```python
from build123d import *

# Parameters (mm, degrees)
CROQUIS1_W              = 300
CROQUIS1_H              = 320
CROQUIS1_W_2            = 280
CROQUIS1_H_2            = 300
SALIENTE_EXTRUIR1_DEPTH = 50
CROQUIS2_R              = 4
CROQUIS2_R_2            = 11
CORTAR_EXTRUIR1_DEPTH   = 321
SKETCH1_R               = 1.09
CUT_EXTRUDE1_DEPTH      = 10


with BuildPart() as part:
    # Croquis1 → Saliente-Extruir1 (new body)
    with BuildSketch(Plane(origin=(0, 0, 0), x_dir=(1, 0, 0), z_dir=(0, 1, 0))):
        Rectangle(CROQUIS1_W, CROQUIS1_H)
        Rectangle(CROQUIS1_W_2, CROQUIS1_H_2, mode=Mode.SUBTRACT)
    extrude(amount=SALIENTE_EXTRUIR1_DEPTH)

    # Croquis2 → Cortar-Extruir1 (cut, through all)
    with BuildSketch(Plane.XY.offset(160)):
        with Locations((-87, 38.5)):
            Circle(CROQUIS2_R)
        with Locations((0, 35.5)):
            Circle(CROQUIS2_R_2)
        with Locations((87, 38.5)):
            Circle(CROQUIS2_R)
    extrude(amount=-CORTAR_EXTRUIR1_DEPTH, mode=Mode.SUBTRACT)

    # Sketch1 → Cut-Extrude1 (cut)
    with BuildSketch(Plane(origin=(0, 0, -160), x_dir=(-1, 0, 0), z_dir=(0, 0, -1))):
        with Locations((0, 13.579689783)):
            Circle(SKETCH1_R)
        with Locations((-21.920310217, 35.5)):
            Circle(SKETCH1_R)
        with Locations((21.920310217, 35.5)):
            Circle(SKETCH1_R)
    extrude(amount=-CUT_EXTRUDE1_DEPTH, mode=Mode.SUBTRACT)


solid = part.part
```
Could you check a few things on this model? Use its own coordinates, in mm. A direction names the side the tool comes from. Round coordinates to 2 decimals unless told otherwise and drop trailing zeros. Loops run counter-clockwise (first coordinate to the right, second up) from the corner with the lowest first, then second, coordinate; pieces in that order, holes last.
Q1. For P1, Ø1.7, axis at x = 0, y = 13.58, coming from the -Z side, with a flat end and sliding along its axis, tell me the tip position at first contact or that it passes through.
Q2. I want a section at B-B (x = -87). Write out the boundary of the cut face in (y, z), and give its area (3 significant figures).
Q3. I want a section at D-D (y = 7). Write out the boundary of the cut face in (x, z), and give its area (3 significant figures).
Q4. On a 3-axis mill with a long thin cutter (end or side, diameter ignored), from which of +Z, -Z, +X, -X, +Y, -Y can I reach the whole of each face in a straight line? I mean faces 5 (the flat face through (-2, 19, 160)), 6 (the flat face through (140, 25, 2)). Say none if no direction works.
Q5. Please list where these lines run through material, in increasing order: L1, parallel to Y at x = 0, z = -153; L2, parallel to X at y = 38.5, z = 93; L3, parallel to Z at x = 110, y = 19.
Q6. Thinking about a two-plate mould opening in Z: for faces 1 (the flat face through (-2, 19, 150)), 2 (the flat face through (150, 25, 2)), 3 (the flat face through (-2, 19, -160)), 4 (the flat face through (-140, 25, 2)), which applies, pulls with the +Z half, pulls with the -Z half, needs draft (parallel to the pull), parting line crosses it, or undercut?
Q7. I want a section at A-A (z = 14). Write out the boundary of the cut face in (x, y).
Q8. I want a section at C-C (x = -125). Write out the boundary of the cut face in (y, z), and give its area (3 significant figures).
Answer below:
1. P1: stops at z = 150
2. outline: (0, -160) - (34.5, -160) - (34.5, -150) - (0, -150) - close; (0, 150) - (34.5, 150) - (34.5, 160) - (0, 160) - close; (42.5, -160) - (50, -160) - (50, -150) - (42.5, -150) - close; (42.5, 150) - (50, 150) - (50, 160) - (42.5, 160) - close
2. area: 840 mm2
3. outline: (-150, -160) - (150, -160) - (150, 160) - (-150, 160) - close; hole (-140, -150) - (140, -150) - (140, 150) - (-140, 150) - close
3. area: 12,000 mm2
4. face 5: +Z, +X, -X, +Y, -Y
4. face 6: +Y, -Y
5. L1: y = 0 to 12.49, 14.67 to 24.5, 46.5 to 50
5. L2: x = -150 to -140, 140 to 150
5. L3: z = -160 to -150, 150 to 160
6. face 1: undercut
6. face 2: needs draft
6. face 3: pulls with the -Z half
6. face 4: undercut
7. outline: (-150, 0) - (-140, 0) - (-140, 50) - (-150, 50) - close; (140, 0) - (150, 0) - (150, 50) - (140, 50) - close
8. outline: (0, -160) - (50, -160) - (50, -150) - (0, -150) - close; (0, 150) - (50, 150) - (50, 160) - (0, 160) - close
8. area: 1,000 mm2
